Check sheet for the modelled part. Datum: model origin and axes. Units: mm. A direction names the side the tool comes from. Round coordinates to 2 decimals unless told otherwise and drop trailing zeros. Loops run counter-clockwise (first coordinate to the right, second up) from the corner with the lowest first, then second, coordinate; pieces in that order, holes last. Notation, with made-up numbers: (13.25, 23) -> (31.25, 23) arc R24 cw to (31.25, 57) -> close; hole circle Ø4 at (22, -25). An arc over 180 degrees is marked (long way). One line per question, with ' | ' between items.
```python
from build123d import *
from build123d.topology import SkipClean

# Parameters (mm, degrees)
SKETCH1_R                = 5.25
SKETCH1_R_2              = 0.53
SKETCH1_R_3              = 1.525
BOSS_EXTRUDE1_DEPTH      = 2
SKETCH2_R                = 3.375
SKETCH2_R_2              = 1.525
BOSS_EXTRUDE2_DEPTH      = 2.5
SKETCH3_R                = 0.8
CUT_EXTRUDE1_DEPTH       = 3.5
BOSS_EXTRUDE3_REACH      = 12.386
BOSS_EXTRUDE3_END_RADIUS = 5.25
SKETCH5_W                = 4.534589286
SKETCH5_H                = 2.5
SKETCH5_R                = 0.8
BOSS_EXTRUDE4_REACH      = 12.386
BOSS_EXTRUDE4_END_RADIUS = 5.25
SKETCH6_W                = 4.534589286
SKETCH6_H                = 2.5
SKETCH6_R                = 0.8
CUT_EXTRUDE2_DEPTH       = 10
CUT_EXTRUDE2_DEPTH_BACK  = 3
SKETCH6_3_R              = 0.8
FILLET1_R                = 0.75
FILLET2_R                = 0.75


with BuildPart() as part:
    # Sketch1 → Boss-Extrude1 (new body)
    with BuildSketch(Plane(origin=(0, 0, 0), x_dir=(1, 0, 0), z_dir=(0, 1, 0))):
        with Locations(Location((0, 0, 0), (0, 0, 270))):
            Circle(SKETCH1_R)
        with Locations(Location((0, 4, 0), (0, 0, 270))):
            Circle(SKETCH1_R_2, mode=Mode.SUBTRACT)
        with Locations(Location((1.530733729, 3.69551813, 0), (0, 0, 270))):
            Circle(SKETCH1_R_2, mode=Mode.SUBTRACT)
        with Locations(Location((2.828427125, 2.828427125, 0), (0, 0, 270))):
            Circle(SKETCH1_R_2, mode=Mode.SUBTRACT)
        with Locations(Location((3.69551813, 1.530733729, 0), (0, 0, 270))):
            Circle(SKETCH1_R_2, mode=Mode.SUBTRACT)
        with Locations(Location((4, 0, 0), (0, 0, 270))):
            Circle(SKETCH1_R_2, mode=Mode.SUBTRACT)
        with Locations(Location((3.69551813, -1.530733729, 0), (0, 0, 270))):
            Circle(SKETCH1_R_2, mode=Mode.SUBTRACT)
        with Locations(Location((2.828427125, -2.828427125, 0), (0, 0, 270))):
            Circle(SKETCH1_R_2, mode=Mode.SUBTRACT)
        with Locations(Location((1.530733729, -3.69551813, 0), (0, 0, 270))):
            Circle(SKETCH1_R_2, mode=Mode.SUBTRACT)
        with Locations(Location((0, -4, 0), (0, 0, 270))):
            Circle(SKETCH1_R_2, mode=Mode.SUBTRACT)
        with Locations(Location((-1.530733729, -3.69551813, 0), (0, 0, 270))):
            Circle(SKETCH1_R_2, mode=Mode.SUBTRACT)
        with Locations(Location((-2.828427125, -2.828427125, 0), (0, 0, 270))):
            Circle(SKETCH1_R_2, mode=Mode.SUBTRACT)
        with Locations(Location((-3.69551813, -1.530733729, 0), (0, 0, 270))):
            Circle(SKETCH1_R_2, mode=Mode.SUBTRACT)
        with Locations(Location((-4, 0, 0), (0, 0, 270))):
            Circle(SKETCH1_R_2, mode=Mode.SUBTRACT)
        with Locations(Location((-3.69551813, 1.530733729, 0), (0, 0, 270))):
            Circle(SKETCH1_R_2, mode=Mode.SUBTRACT)
        with Locations(Location((-2.828427125, 2.828427125, 0), (0, 0, 270))):
            Circle(SKETCH1_R_2, mode=Mode.SUBTRACT)
        with Locations(Location((-1.530733729, 3.69551813, 0), (0, 0, 270))):
            Circle(SKETCH1_R_2, mode=Mode.SUBTRACT)
        with Locations(Location((0, 0, 0), (0, 0, 270))):
            Circle(SKETCH1_R_3, mode=Mode.SUBTRACT)
    extrude(amount=BOSS_EXTRUDE1_DEPTH)

    # Sketch2 → Boss-Extrude2 (add)
    with BuildSketch(Plane(origin=(0, 2, 0), x_dir=(1, 0, 0), z_dir=(0, 1, 0))):
        with Locations(Location((0, 0, 0), (0, 0, 270))):
            Circle(SKETCH2_R)
        with Locations(Location((0, 0, 0), (0, 0, 270))):
            Circle(SKETCH2_R_2, mode=Mode.SUBTRACT)
    extrude(amount=BOSS_EXTRUDE2_DEPTH)

    # Sketch3 → Cut-Extrude1 (cut)
    with BuildSketch(Plane.XY):
        with Locations(Location((0, 3, 0), (0, 0, 90))):
            Circle(SKETCH3_R)
    extrude(amount=-CUT_EXTRUDE1_DEPTH, mode=Mode.SUBTRACT)

    # Boss-Extrude3: up to this cylinder (the profile starts inside it)
    with SkipClean():  # the faces are left unmerged after this step: merging them gives an invalid solid
        boss_extrude3_end = Plane(origin=(0, 2.051781, 0), z_dir=(0, -1, 0)) * Cylinder(BOSS_EXTRUDE3_END_RADIUS, 36.272, mode=Mode.PRIVATE)
        # Sketch5 → Boss-Extrude3 (add, up to the surface)
        with BuildSketch(Plane.XY.offset(-2.5), mode=Mode.PRIVATE) as boss_extrude3_sk1:
            with Locations((0, 3.25)):
                Rectangle(SKETCH5_W, SKETCH5_H)
            with Locations((0, 3)):
                Circle(SKETCH5_R, mode=Mode.SUBTRACT)
        boss_extrude3_tool1 = extrude(boss_extrude3_sk1.sketch, amount=-BOSS_EXTRUDE3_REACH, mode=Mode.PRIVATE) & boss_extrude3_end
        add(boss_extrude3_tool1.solids().sort_by_distance((0, 2.051781, -2.5))[0])

    # Boss-Extrude4: up to this cylinder (the profile starts inside it)
    with SkipClean():  # the faces are left unmerged after this step: merging them gives an invalid solid
        boss_extrude4_end = Plane(origin=(0, 3.25, 0), z_dir=(0, -1, 0)) * Cylinder(BOSS_EXTRUDE4_END_RADIUS, 36.272, mode=Mode.PRIVATE)
        # Sketch6 → Boss-Extrude4 (add, up to the surface)
        with BuildSketch(Plane(origin=(2.5, 0, 0), x_dir=(0, 0, -1), z_dir=(1, 0, 0)), mode=Mode.PRIVATE) as boss_extrude4_sk1:
            with Locations((0, 3.25)):
                Rectangle(SKETCH6_W, SKETCH6_H)
            with Locations(Location((0, 3, 0), (0, 0, 180))):
                Circle(SKETCH6_R, mode=Mode.SUBTRACT)
        boss_extrude4_tool1 = extrude(boss_extrude4_sk1.sketch, amount=BOSS_EXTRUDE4_REACH, mode=Mode.PRIVATE) & boss_extrude4_end
        add(boss_extrude4_tool1.solids().sort_by_distance((2.5, 3.25, 2.215514))[0])

    # Sketch6<3> → Cut-Extrude2 (cut, two sides: drawn at the far end of the back side and taken through both)
    with SkipClean():  # the faces are left unmerged after this step: merging them gives an invalid solid
        with BuildSketch(Plane(origin=(2.5, 0, 0), x_dir=(0, 0, -1), z_dir=(1, 0, 0)).offset(-CUT_EXTRUDE2_DEPTH_BACK)):
            with Locations(Location((0, 3, 0), (0, 0, 180))):
                Circle(SKETCH6_3_R)
        extrude(amount=CUT_EXTRUDE2_DEPTH + CUT_EXTRUDE2_DEPTH_BACK, mode=Mode.SUBTRACT)

    # Fillet1
    fillet1_edges = [part.edges().sort_by_distance(p)[0] for p in [
        (2.267294643, 3.25, -4.735174231),
        (-2.267294643, 3.25, -4.735174231),
        (4.735174231, 3.25, 2.267294643),
        (4.735174231, 3.25, -2.267294643),
    ]]
    fillet(fillet1_edges, radius=FILLET1_R)

    # Fillet2
    # the kernel refuses this fillet: 0.75 mm, written as the material it adds along each edge
    with BuildSketch(Plane(origin=(2.267294643, 4.5, -2.5), x_dir=(0, 0, -1), z_dir=(0, -1, 0))) as fillet2_piece_1:
        with BuildLine():
            CenterArc((0.312749195, 0.75), FILLET2_R, 227.009382104, 42.990617896)
            ThreePointArc((-0.198659749, 0.201400974), (-0.09721877, 0.102782858), (0, 0))
            Line((0, 0), (0.312749195, 0))
        make_face()
    extrude(amount=3.281872988)
    with BuildSketch(Plane(origin=(-2.267294643, 1.218127012, -2.5), x_dir=(-0.7119351792170611, 0, 0.7022451855250923), z_dir=(0, 1, 0))) as fillet2_piece_2:
        with BuildLine():
            CenterArc((0.314324768, -0.749341043), FILLET2_R, 92.40196785, 42.990617896)
            Line((-0.219626617, -0.222657154), (0, 0))
            ThreePointArc((0, 0), (0.141446146, -0.002965304), (0.282892291, 0))
        make_face()
    extrude(amount=3.281872988)
    with BuildSketch(Plane(origin=(2.5, 1.218127012, 2.267294643), x_dir=(1, 0, 0), z_dir=(0, 1, 0))) as fillet2_piece_3:
        with BuildLine():
            CenterArc((0.312749195, -0.75), FILLET2_R, 90, 42.990617896)
            ThreePointArc((-0.198659749, -0.201400974), (-0.09721877, -0.102782858), (0, 0))
            Line((0, 0), (0.312749195, 0))
        make_face()
    extrude(amount=3.281872988)
    with BuildSketch(Plane(origin=(2.5, 4.5, -2.267294643), x_dir=(-0.7022451855250915, 0, -0.7119351792170617), z_dir=(0, -1, 0))) as fillet2_piece_4:
        with BuildLine():
            CenterArc((0.314324768, 0.749341043), FILLET2_R, 224.607414254, 42.990617896)
            Line((-0.219626617, 0.222657154), (0, 0))
            ThreePointArc((0, 0), (0.141446146, 0.002965304), (0.282892291, 0))
        make_face()
    extrude(amount=3.281872988)


solid = part.part
```
(1) Mould release check, pull along Z, two halves, no side actions. Record for faces 1 (the face through (3.7, 2, 1.5)), 2 (the face through (3.2, 2, -3.4)), 3 (the face through (-2.44, 3.23, 2.33)), 4 (the face through (3.855, 0.986, -1.025)): +Z half, -Z half, draft (parallel to the pull), parting line (faces both ways), or undercut.
Answer:
face 1: undercut | face 2: draft | face 3: parting line | face 4: undercut
(2) Sectioned sample at D-D, the plane z = -4. Record the cut outline in (x, y).
Answer:
outline: (-3.4, 0) -> (-1.96, 0) -> (-1.96, 2) -> (-1.1, 2) -> (-1.1, 0) -> (-0.53, 0) -> (-0.53, 2) -> (0.53, 2) -> (0.53, 0) -> (1.1, 0) -> (1.1, 2) -> (1.96, 2) -> (1.96, 0) -> (3.4, 0) -> (3.4, 2) -> (2.27, 2) -> (2.27, 4.5) -> (-2.27, 4.5) -> (-2.27, 2) -> (-3.4, 2) -> close; hole circle Ø1.6 at (0, 3)
(3) Sectioned sample at B-B, the plane z = 0. Record the cut outline in (x, y) (3 decimals).
Answer:
outline: (-5.25, 0) -> (-4.53, 0) -> (-4.53, 2) -> (-5.25, 2) -> close; (-3.47, 0) -> (-1.525, 0) -> (-1.525, 4.5) -> (-3.375, 4.5) -> (-3.375, 2) -> (-3.47, 2) -> close; (1.525, 0) -> (3.47, 0) -> (3.47, 2) -> (4.53, 2) -> (4.53, 0) -> (5.25, 0) -> (5.25, 2.2) -> (1.525, 2.2) -> close; (1.525, 3.8) -> (5.25, 3.8) -> (5.25, 4.5) -> (1.525, 4.5) -> close
(4) Sectioned sample at C-C, the plane x = 4. Record the cut outline in (y, z), and give its area (3 significant figures).
Answer:
outline: (0, -3.4) -> (2, -3.4) -> (2, -2.27) -> (4.5, -2.27) -> (4.5, 2.27) -> (2, 2.27) -> (2, 3.4) -> (0, 3.4) -> (0, 1.96) -> (2, 1.96) -> (2, 1.1) -> (0, 1.1) -> (0, 0.53) -> (2, 0.53) -> (2, -0.53) -> (0, -0.53) -> (0, -1.1) -> (2, -1.1) -> (2, -1.96) -> (0, -1.96) -> close; hole circle Ø1.6 at (3, 0) | area: 17.3 mm2
(5) Sectioned sample at A-A, the plane y = 3. Record the cut outline in (x, z) (3 decimals).
Answer:
outline: (-2.469, -2.301) arc R0.75 cw to (-2.267, -2.813) -> (-2.267, -4.236) arc R0.75 ccw to (-1.77, -4.943) arc R5.25 ccw to (-0.8, -5.189) -> (-0.8, -1.298) arc R1.525 cw (long way) to (1.298, 0.8) -> (5.189, 0.8) arc R5.25 ccw to (4.943, 1.77) arc R0.75 ccw to (4.236, 2.267) -> (2.813, 2.267) arc R0.75 cw to (2.301, 2.469) arc R3.375 ccw to start; (0.8, -5.189) arc R5.25 ccw to (1.77, -4.943) arc R0.75 ccw to (2.267, -4.236) -> (2.267, -2.813) arc R0.75 cw to (2.395, -2.395) arc R0.75 cw to (2.813, -2.267) -> (4.236, -2.267) arc R0.75 ccw to (4.943, -1.77) arc R5.25 ccw to (5.189, -0.8) -> (1.298, -0.8) arc R1.525 cw to (0.8, -1.298) -> close
(6) Scan lines: probe 1 along X at (y, z) = (1.8, 0) (3 decimals); probe 2 along Z at (x, y) = (3, 1.6); probe 3 along X at (y, z) = (4.1, 0.5). Record each from-to range of solid material in increasing order.
Answer:
probe 1: x = -5.25 to -4.53, -3.47 to -1.525, 1.525 to 3.47, 4.53 to 5.25 | probe 2: z = -4.31 to -3.33, -2.33 to 2.33, 3.33 to 4.31 | probe 3: x = -3.34 to -1.44, 1.44 to 5.23
(7) Go/stop test with flat-tipped pins: pin 1 (0.8 mm diameter, centred on x = -2.83, z = 2.83, fed in from -Y); pin 2 (0.8 mm diameter, centred on x = 0, z = -4, fed in from -Y). Record where each tip stops, or that it passes through.
Answer:
pin 1: passes through | pin 2: stops at y = 2
(8) Set-up check for faces 5 (the face through (4, 2, 0)), 6 (the face through (-2.267, 3, -4)), 7 (the face through (4, 3, -2.267)), 8 (the face through (1.2, 4.5, -1.2)): record each of +Z, -Z, +X, -X, +Y, -Y from which the full face is reachable in a straight line by a thin tool's end or side.
Answer:
face 5: -Y | face 6: -Z, -X, +Y | face 7: -Z, +X, +Y | face 8: +Z, -Z, +X, -X, +Y
